For this review, take the finished solid that the model builds, in its own axes (mm). Face numbers are marked on the shaded views. A direction names the side the tool comes from. Give positions to 0.01 mm unless a question says otherwise; leave off trailing zeros. Loops run counter-clockwise (first coordinate to the right, second up) from the corner with the lowest first, then second, coordinate; pieces in that order, holes last. Notation, with made-up numbers: (51, -36) -> (94, -36) arc R19 cw to (94, -8) -> close; hole circle Ø6 at (77, 29). An arc over 180 degrees is marked (long way). Answer as CSV lines item,"result". Start each with the question number.
Item 1: For L1, parallel to X at y = 6.95, z = 0; L2, parallel to Z at x = 2.5, y = 6.75; L3, parallel to Y at x = -1, z = -1.75, list the stretches that pass through material, from the lowest coordinate up. Write a range as from..to.
Item 2: Clearance check with flat-ended pins moving along their axes: P1, Ø5, axis at y = 7.5, z = -1.5, coming from the -X side; P2, Ø2, axis at y = 4, z = 5.5, coming from the -X side; P3, Ø2, axis at x = -5.5, z = 2, coming from the +Y side. State where each tip first meets the part, or that it passes through.
Item 3: Add section C-C on y = 2.5. State the section outline as (x, z) points (3 decimals), plus the area to 3 significant figures.
Item 4: The part is to be moulded in two halves that separate along Z. For the marked faces 1, 2 and 3, say which applies: +Z half, -Z half, draft (parallel to the pull), parting line (faces both ways), or undercut.
Item 5: Add section B-B on z = 0. State the section outline as (x, y) points (1 decimal), plus the area to 3 significant figures.
Item 6: Machinability: for the marked faces 4 and 5, which of the approach directions +Z, -Z, +X, -X, +Y, -Y give a long, thin tool a straight path to every point of the face, cutting with its end or side? Answer none if there is none.
Item 7: Add section A-A on x = 0. State the section outline as (y, z) points (1 decimal), plus the area to 3 significant figures.
```python
from build123d import *

# Parameters (mm, degrees)
F3_R      = 1.85
F4_DEPTH  = 7
F5_R      = 1.2
F6_DEPTH  = 2
F8_DEPTH  = 4.5
F9_R      = 1
F10_R     = 1.2
F11_DEPTH = 4.5
F12_R     = 5


with BuildPart() as f1:
    # F0 (on Top) → F1 (revolve)
    with BuildSketch(Plane.XY):
        with BuildLine():
            Line((0, 9), (0, 0))
            Line((0, 0), (11, 0))
            Line((11, 0), (11, 4))
            Line((11, 4), (10.5, 7))
            ThreePointArc((10.5, 7), (10.0017468007, 7.1915925315), (9.5, 7.3738398822))
            Line((9.5, 7.3738398822), (9.5, 6.5449972332))
            Line((9.5, 6.5449972332), (9, 6.5449972332))
            Line((9, 6.5449972332), (9, 7.5449972332))
            ThreePointArc((9, 7.5449972332), (4.5584271698, 8.6339031037), (0, 9))
        make_face()
    revolve(axis=Axis((0, 4.5, 0), (0, 1, 0)))

    # F3 (on offset) → F4 (cut)
    with BuildSketch(Plane.XZ.offset(-9)):
        with Locations((6.65, 4.625)):
            Circle(F3_R)
    extrude(amount=F4_DEPTH, mode=Mode.SUBTRACT)

    # F5 (on face) → F6 (cut, through all)
    with BuildSketch(Plane(origin=(0, 2, 0), x_dir=(-1, 0, 0), z_dir=(0, 1, 0))):
        with Locations((-6.65, 4.625)):
            Circle(F5_R)
    extrude(amount=-F6_DEPTH, mode=Mode.SUBTRACT)

    # F7 (on offset) → F8 (cut)
    with BuildSketch(Plane.XZ.offset(-9)):
        with BuildLine():
            Line((4.9918584287, -4.0461524227), (-3.38657071, 10.4657125331))
            ThreePointArc((-3.38657071, 10.4657125331), (-8.661662033, 6.780531751), (-10.9726648996, 0.775))
            Line((-10.9726648996, 0.775), (-3.1032576969, 0.775))
            Line((-3.1032576969, 0.775), (1.0081415713, -6.3461524227))
            Line((1.0081415713, -6.3461524227), (4.9918584287, -4.0461524227))
        make_face()
    extrude(amount=F8_DEPTH, mode=Mode.SUBTRACT)

    # F9
    f9_edges = [f1.edges().sort_by_distance(p)[0] for p in [
        (4.991858, 6.383907, -4.046152),
        (1.008142, 6.383907, -6.346152),
    ]]
    fillet(f9_edges, radius=F9_R)

    # F10 (on face) → F11 (cut, through all)
    with BuildSketch(Plane(origin=(0, 4.5, 0), x_dir=(-1, 0, 0), z_dir=(0, 1, 0))):
        with Locations((6.65, 4.625)):
            Circle(F10_R)
    extrude(amount=-F11_DEPTH, mode=Mode.SUBTRACT)

    # F12
    f12_edges = [f1.edges().sort_by_distance(p)[0] for p in [
        (-3.103258, 6.66017, 0.775),
    ]]
    fillet(f12_edges, radius=F12_R)


solid = f1.part
```
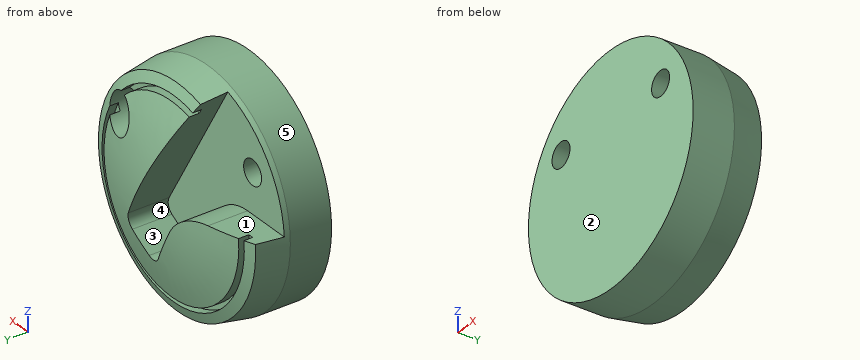
Computed values:
1,L1,"-10.51..-9.5, -9..-3.32, 2.66..9, 9.5..10.51"
1,L2,"-10.24..-9.17, -8.65..-5.48, 0.27..8.65, 9.17..10.24"
1,L3,"0..4.5"
2,P1,"x = -10.79"
2,P2,"x = -10.04"
2,P3,"y = 4.5"
3,outline,"circle Ø22 at (0, 0); hole circle Ø2.4 at (-6.65, 4.625); hole circle Ø3.7 at (6.65, 4.625)"
3,area,"365 mm²"
4,face 1,"+Z half"
4,face 2,"draft"
4,face 3,"undercut"
5,outline,"(-11, 0) -> (11, 0) -> (11, 4) -> (10.5, 7) arc R28.6 ccw to (9.5, 7.4) -> (9.5, 6.5) -> (9, 6.5) -> (9, 7.5) arc R28.6 ccw to (2.7, 8.9) -> (2.7, 4.5) -> (-3.3, 4.5) -> (-3.3, 8.8) arc R28.6 ccw to (-9, 7.5) -> (-9, 6.5) -> (-9.5, 6.5) -> (-9.5, 7.4) arc R28.6 ccw to (-10.5, 7) -> (-11, 4) -> close"
5,area,"153 mm²"
6,face 4,"+Y"
6,face 5,"+Y, -Y"
7,outline,"(0, -11) -> (4, -11) -> (7, -10.5) arc R28.6 ccw to (7.4, -9.5) -> (6.5, -9.5) -> (6.5, -9) -> (7.5, -9) arc R28.6 ccw to (8.6, -4.6) -> (4.5, -4.6) -> (4.5, 4.6) -> (8.6, 4.6) arc R28.6 ccw to (7.5, 9) -> (6.5, 9) -> (6.5, 9.5) -> (7.4, 9.5) arc R28.6 ccw to (7, 10.5) -> (4, 11) -> (0, 11) -> close"
7,area,"140 mm²"
